The figure shows three views and two pictorial views of one solid part (mm, origin at its lowest corner). Answer the questions. A direction names the side the tool comes from. Round coordinates to 2 decimals unless told otherwise and drop trailing zeros. Write each loop counter-clockwise with the first axis right and the second up, starting at its lowest first coordinate (ties: lowest second). Pieces come first, ordered by that corner, then holes.
Item 1: Find section B-B on z = 0.65. Give the vertices of the cut face in (x, y), then the cut area to 3 significant figures.
Item 2: Find section D-D on x = 2.75. Give the vertices of the cut face in (y, z), then the cut area to 3 significant figures.
Item 3: Find section A-A on y = 1.5. Give the vertices of the cut face in (x, z).
Item 4: This flat-tipped pin is pushed along its axis until it touches: pin 1 (0.9 mm diameter, centred on y = 2, z = 2, fed in from -X). Where does it stop, or does it pass through?
Item 5: A tool of negligible diameter and unlimited length cuts with its end or side. For the marked faces 1, 2 and 3, from which of +Z, -Z, +X, -X, +Y, -Y can it reach the whole face along a straight path? Write none if from no direction.
Item 6: Find the intervals of material crossed by probe 1 along X at (y, z) = (1.6, 0.2); probe 2 along Y at (x, z) = (1.25, 1.4); probe 3 along Y at (x, z) = (8.75, 0.7), in increasing order.
Item 7: Find section C-C on x = 6.5. Give the vertices of the cut face in (y, z).
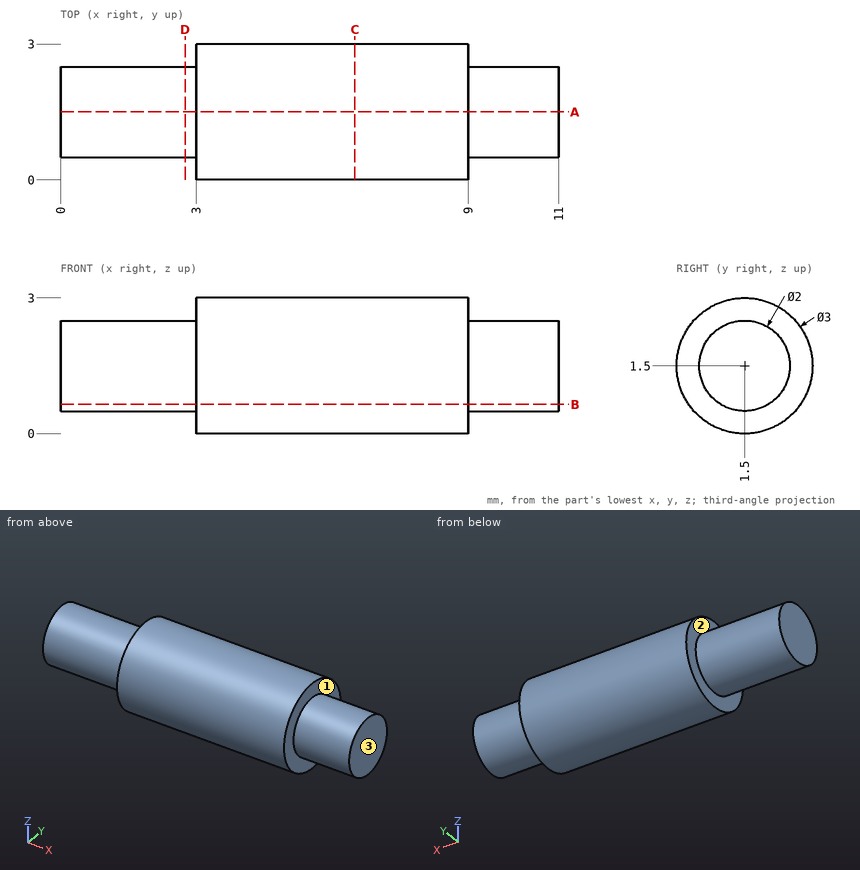
Check values:
1. outline: (0, 0.97) - (3, 0.97) - (3, 0.26) - (9, 0.26) - (9, 0.97) - (11, 0.97) - (11, 2.03) - (9, 2.03) - (9, 2.74) - (3, 2.74) - (3, 2.03) - (0, 2.03) - close
1. area: 20.1 mm2
2. outline: circle Ø2 at (1.5, 1.5)
2. area: 3.14 mm2
3. outline: (0, 0.5) - (3, 0.5) - (3, 0) - (9, 0) - (9, 0.5) - (11, 0.5) - (11, 2.5) - (9, 2.5) - (9, 3) - (3, 3) - (3, 2.5) - (0, 2.5) - close
4. pin 1: stops at x = 0
5. face 1: +X
5. face 2: -X
5. face 3: +Z, -Z, +X, +Y, -Y
6. probe 1: x = 3 to 9
6. probe 2: y = 0.51 to 2.49
6. probe 3: y = 0.23 to 2.77
7. outline: circle Ø3 at (1.5, 1.5)
